For this review, take the finished solid that the model builds, in its own axes (mm). Give positions to 0.01 mm unless a question says otherwise; leave off trailing zeros. Loops run counter-clockwise (first coordinate to the right, second up) from the corner with the lowest first, then second, coordinate; pieces in that order, holes last.
Autodesk Inventor part; units mm, degrees
ref_plane "YZ Plane" through (0, 0, 0) normal (1, 0, 0) x (0, 1, 0)
ref_plane "XZ Plane" through (0, 0, 0) normal (0, 1, 0) x (-1, 0, 0)
ref_plane "XY Plane" through (0, 0, 0) normal (0, 0, 1) x (1, 0, 0)
sketch "Sketch1" plane through (0, 0, 0) normal (0, 0, 1) x (1, 0, 0)
  line L0 (315, -9.5) -> (-315, -9.5)
  line L1 (-315, -9.5) -> (-315, 9.5)
  line L2 (-315, 9.5) -> (315, 9.5)
  line L3 (315, 9.5) -> (315, -9.5)
  line L4 (315, -9.5) -> (-315, 9.5) construction
  line L5 (-315, -9.5) -> (315, 9.5) construction
  point P0 (0, 0)
  dimension "d0" = 630
  dimension "d1" = 19
extrude "Extrusion1" add sketch "Sketch1" along normal blind 15
sketch "Sketch2" plane through (-315, 9.5, 0) normal (0, 1, 0) x (1, 0, 0)
  line L0 (630, 0) -> (0, 0)
  line L1 (0, 0) -> (15, -15)
  line L2 (630, -15) -> (0, -15)
  line L3 (15, -15) -> (0, -15)
  line L4 (0, -15) -> (0, 0)
  point P0 (315, 0)
  dimension "d4" = 45
extrude "Extrusion2" cut sketch "Sketch2" against normal through all
mirror "Mirror1" about plane through (0, 0, 0) normal (1, 0, 0) of "Extrusion2"
ref_plane "Work Plane1" through (0, 0, 0) normal (1, 0, 0) x (0, 1, 0)
properties part number "lengthBinding"
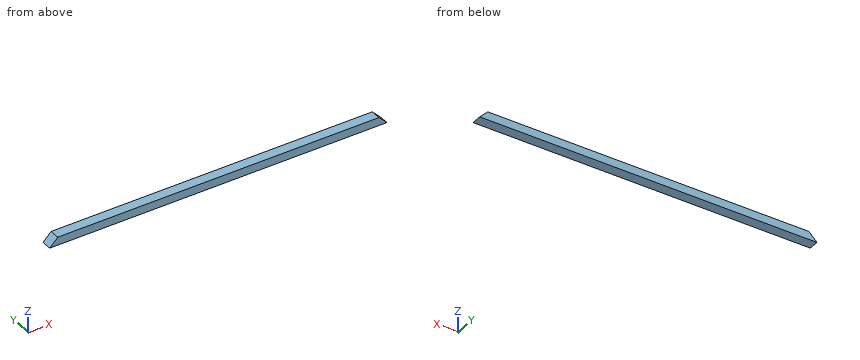
Item 1: Take a section at B-B on y = 0. Give the boundary of the cut face in (x, z), and give its area (4 significant figures).
Answer:
outline: (-315, 0) - (315, 0) - (300, 15) - (-300, 15) - close
area: 9,225 mm2
Item 2: For L1, parallel to X at y = 0, z = 1.25; L2, parallel to X at y = -6, z = 5.5, list the stretches that pass through material, from the lowest coordinate up.
Answer:
L1: x = -313.75 to 313.75
L2: x = -309.5 to 309.5
Item 3: Clearance check with flat-ended pins moving along their axes: pin 1 Ø8 at (y, z) = (-4.5, 11) entering from -X; pin 2 Ø8 at (y, z) = (-6.5, 12.5) entering from +X. State where each tip first meets the part, or that it passes through.
Answer:
pin 1: stops at x = -308
pin 2: stops at x = 306.5
Item 4: Take a section at A-A on z = 10.75. Give the boundary of the cut face in (x, y), and give its area (3 significant figures).
Answer:
outline: (-304.25, -9.5) - (304.25, -9.5) - (304.25, 9.5) - (-304.25, 9.5) - close
area: 11,600 mm2
